Geometry: final body of the model. Coordinates: model frame, mm. Face numbers are marked on the shaded views. A direction names the side the tool comes from. Coordinates: 2 decimals unless noted, no trailing zeros. Order: outer loops, then holes, each group sorted by start corner. A loop starts at its lowest first (then second) coordinate and runs counter-clockwise, first axis right, second up. Notation, with made-up numbers: M 66,76.5 L 112,76.5 A27 ccw 112,109.5 Z; hole C -22,67.5 d4. An arc over 180 degrees is marked long. Use CSV: the item, a comma, the result in double quotes. Start each with the question number.
1. Pull-direction query (X, two-part tool) for the marked faces 4, 5, 6 and 7; classes: pulls with the +X half, pulls with the -X half, needs draft (parallel to the pull), parting line crosses it, or undercut.
2. Material intervals for line 1 (Z direction, x = -11, y = -30) (3 decimals); line 2 (Z direction, x = 104, y = -31.5) (3 decimals); line 3 (Y direction, x = 51.5, z = 52), sorted ascending.
3. Section query A-A on z = 0.5. Return the cut outline in (x, y) (3 decimals), and give its area (3 significant figures).
4. Section query C-C on x = 136. Return the cut outline in (y, z) (3 decimals).
5. Section query B-B on y = 42. Return the cut outline in (x, z) (3 decimals), and give its area (3 significant figures).
6. Set-up query: the marked faces 1, 2 and 3. Return all of +Z, -Z, +X, -X, +Y, -Y with unobstructed straight access to the full face (end or side cutting, diameter ignored); none if empty.
7. First-contact query: P1, Ø10, axis at x = -5, z = 25.5, coming from the +Y side; P2, Ø10, axis at x = 100.5, y = -35.5, coming from the -Z side; P3, Ø21.5, axis at x = 48, z = 44.5, coming from the -Y side. Flat tips, straight axial feed; report the tip coordinate or a pass-through.
8. Section query D-D on y = 11. Return the cut outline in (x, z) (3 decimals), and give its area (3 significant figures).
from build123d import *

# Parameters (mm, degrees)
F1_DEPTH = 63.5
F2_DEPTH = 25.4
F3_DEPTH = 7.9375
F5_R     = 6.35


with BuildPart() as f1:
    # F0 (on Front) → F1 (new body, symmetric)
    with BuildSketch(Plane.XZ):
        Polygon((23.849781, 9.525), (-41.275, 9.525), (-41.275, -9.525), (41.275, -9.525), (41.275, 9.525), align=None)
    extrude(amount=F1_DEPTH, both=True)

    # F0 (on Front) → F2 (join, symmetric)
    with BuildSketch(Plane.XZ):
        with BuildLine():
            Line((23.849781, 23.8252), (23.849781, 9.525))
            Line((23.849781, 9.525), (41.275, 9.525))
            Line((41.275, 9.525), (41.275, 23.8252))
            ThreePointArc((41.275, 23.8252), (46.854616, 37.295584), (60.325, 42.8752))
            Line((60.325, 42.8752), (60.325, 60.300419))
            ThreePointArc((60.325, 60.300419), (34.533125, 49.617075), (23.849781, 23.8252))
        make_face()
        Polygon((60.325, 66.675), (60.325, 60.300419), (60.325, 42.8752), (60.325, 38.1), (111.125, 38.1), (111.125, 66.675), align=None)
    extrude(amount=F2_DEPTH, both=True)

    # F0 (on Front) → F3 (join, symmetric)
    with BuildSketch(Plane.XZ):
        with BuildLine():
            add(Edge.make_bspline(
                [(-41.275, 9.525), (-39.523579, 39.352842), (10.464912, 63.553624), (60.325, 60.300419)],
                knots=[0, 0, 0, 0, 113.581263, 113.581263, 113.581263, 113.581263], degree=3))
            Line((-41.275, 9.525), (23.849781, 9.525))
            Line((23.849781, 9.525), (23.849781, 23.8252))
            ThreePointArc((23.849781, 23.8252), (34.533125, 49.617075), (60.325, 60.300419))
        make_face()
    extrude(amount=F3_DEPTH, both=True)

    # F0 (on Front) → F4 (revolve)
    with BuildSketch(Plane.XZ):
        Polygon((60.325, 66.675), (60.325, 60.300419), (60.325, 42.8752), (60.325, 38.1), (111.125, 38.1), (111.125, 66.675), align=None)
    revolve(axis=Axis((111.125, 0, 52.3875), (0, 0, 1)))

    # F5
    f5_edges = [f1.edges().sort_by_distance(p)[0] for p in [
        (41.275, -63.5, 0),
        (-41.275, -63.5, 0),
        (41.275, 63.5, 0),
        (-41.275, 63.5, 0),
    ]]
    fillet(f5_edges, radius=F5_R)


solid = f1.part
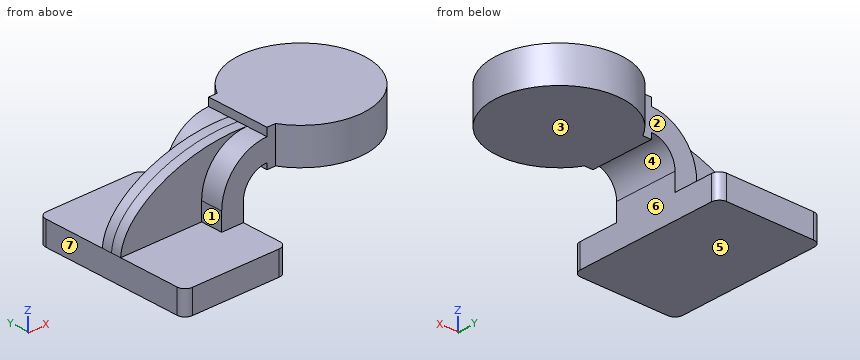
Results list:
1,face 4,"undercut"
1,face 5,"needs draft"
1,face 6,"pulls with the +X half"
1,face 7,"pulls with the -X half"
2,line 1,"z = -9.525 to 9.525"
2,line 2,"z = 38.1 to 66.675"
2,line 3,"y = -25.4 to 25.4"
3,outline,"M -41.275,-57.15 A6.35 ccw -34.925,-63.5 L 34.925,-63.5 A6.35 ccw 41.275,-57.15 L 41.275,57.15 A6.35 ccw 34.925,63.5 L -34.925,63.5 A6.35 ccw -41.275,57.15 Z"
3,area,"10,400 mm²"
4,outline,"M -44.293,38.1 L 44.293,38.1 L 44.293,66.675 L -44.293,66.675 Z"
5,outline,"M -41.275,-9.525 L 41.275,-9.525 L 41.275,9.525 L -41.275,9.525 Z; M 82.548,38.1 L 139.702,38.1 L 139.702,66.675 L 82.548,66.675 Z"
5,area,"3,210 mm²"
6,face 1,"+Z, -X, -Y"
6,face 2,"+Z, -X, +Y"
6,face 3,"-Z, +X, +Y, -Y"
7,P1,"stops at y = 7.94"
7,P2,"stops at z = 38.1"
7,P3,"stops at y = -25.4"
8,outline,"M -41.275,-9.525 L 41.275,-9.525 L 41.275,23.825 A19.05 cw 60.325,42.875 L 60.325,38.1 L 160.72,38.1 L 160.72,66.675 L 60.325,66.675 L 60.325,60.3 A36.475 ccw 23.85,23.825 L 23.85,9.525 L -41.275,9.525 Z"
8,area,"5,450 mm²"
